```python
from build123d import *

# Parameters (mm, degrees)
SKETCH2_R           = 12.5
SKETCH2_R_2         = 11.5
SKETCH14_W          = 50
SKETCH14_H          = 23
BOSS_EXTRUDE1_DEPTH = 381.5
SKETCH15_R          = 6.5
CUT_EXTRUDE1_DEPTH  = 436.5
SKETCH16_W          = 40
SKETCH16_H          = 100
BOSS_EXTRUDE2_DEPTH = 5
SKETCH18_R          = 6.5
BOSS_EXTRUDE3_DEPTH = 10


with BuildPart() as part:
    # Sweep-Thin1: sweep along a path in Sketch1
    with BuildLine(Plane(origin=(0, 0, 0), x_dir=(1, 0, 0), z_dir=(0, 1, 0))) as sweep_thin1_path:
        Line((0, 395), (-610, 395))
        ThreePointArc((-610, 395), (-716.066017178, 351.066017178), (-760, 245))
        Line((-760, 245), (-760, -245))
        ThreePointArc((-760, -245), (-716.066017178, -351.066017178), (-610, -395))
        Line((-610, -395), (0, -395))
    # Sketch2 → Sweep-Thin1 (sweep)
    with BuildSketch(Plane(origin=(0, 0, 395), x_dir=(0, 0, -1), z_dir=(1, 0, 0))):
        with Locations((12.5, 0)):
            Circle(SKETCH2_R)
        with Locations((12.5, 0)):
            Circle(SKETCH2_R_2, mode=Mode.SUBTRACT)
    sweep(path=sweep_thin1_path.line)

    # Sketch14 → Boss-Extrude1 (add, symmetric)
    with BuildSketch(Plane.XY):
        with Locations((-75, 0)):
            Rectangle(SKETCH14_W, SKETCH14_H)
    extrude(amount=BOSS_EXTRUDE1_DEPTH, both=True)

    # Sketch15 → Cut-Extrude1 (cut, symmetric)
    with BuildSketch(Plane.XY):
        with Locations((-15, 0)):
            Circle(SKETCH15_R)
    extrude(amount=CUT_EXTRUDE1_DEPTH, both=True, mode=Mode.SUBTRACT)

    # Sketch16 → Boss-Extrude2 (add)
    with BuildSketch(Plane.XZ.offset(11.5)):
        with Locations((-75, -307.601020514)):
            Rectangle(SKETCH16_W, SKETCH16_H)
    extrude(amount=BOSS_EXTRUDE2_DEPTH)

    # Sketch18 → Boss-Extrude3 (add)
    with BuildSketch(Plane(origin=(0, 0, -317.601020514), x_dir=(-1, 0, 0), z_dir=(0, 0, -1))):
        with BuildLine():
            Line((90, -16.5), (60, -16.5))
            Line((60, -16.5), (198.241047903, -193.477674036))
            ThreePointArc((198.241047903, -193.477674036), (204.902077591, -197.247200167), (212.277594342, -195.202598394))
            Line((212.277594342, -195.202598394), (220.426068509, -188.837650874))
            ThreePointArc((220.426068509, -188.837650874), (224.214109013, -182.01512928), (221.946736533, -174.548197259))
            Line((221.946736533, -174.548197259), (90, -16.5))
        make_face()
        with Locations((204.040209344, -176.258653836)):
            Circle(SKETCH18_R, mode=Mode.SUBTRACT)
    boss_extrude3 = extrude(amount=BOSS_EXTRUDE3_DEPTH)

    # Mirror1: Boss-Extrude3 across plane
    add(boss_extrude3.mirror(Plane(origin=(0, 0, -302.601020514), x_dir=(1, 0, 0), z_dir=(0, 0, -1))))


solid = part.part
```
Geometry check sheet. Reference: the model listing, model coordinates, mm. A direction names the side the tool comes from. Coordinates: 2 decimals unless noted, no trailing zeros. Loops run counter-clockwise (first coordinate to the right, second up) from the corner with the lowest first, then second, coordinate; pieces in that order, holes last. Notation, with made-up numbers: (40, 4) - (68, 4) arc R25 cw to (68, 23) - close; hole circle Ø8 at (66, 13). An arc over 180 degrees is marked (long way). One line per item, written item: value. Start each with the question number.
(1) Material ranges on line 1 (Z direction, x = -277, y = 0); line 2 (Z direction, x = -90.5, y = -55); line 3 (Y direction, x = -244, z = -382), recorded low to high. Write a range as [from, to].
(2) Depth check by flat-ended pin: P1, Ø1.5, axis at x = -76, y = -13.5, coming from the -Z side; P2, Ø8, axis at x = -96.5, z = -251, coming from the -Y side; P3, Ø12, axis at x = -114, z = -280.5, coming from the +Y side. Enter the tip coordinate at first touch or a pass-through.
(3) Cross-section at C-C on x = -601. Enter the section's corners in (y, z).
(4) Cross-section at B-B on y = -112.5. Enter the section's corners in (x, z).
(5) Cross-section at D-D on y = -47. Enter the section's corners in (x, z), plus the area to 3 significant figures.
(6) Cross-section at A-A on z = -137. Enter the section's corners in (x, y).
(7) Mould release check, pull along Y, two halves, no side actions. Record for faces 1 (the cylindrical face through (-300.73, 0.51, 393.99)), 2 (the cylindrical face through (-309.27, 3.755, -370.577)), 3 (the flat face through (-148, -106, -317.601)): released by +Y, released by -Y, zero draft, split by the parting line, or undercut.
(8) Tool access check on faces 4 (the flat face through (-148, -106, -327.601)), 5 (the flat face through (-50, 0, 5)), 6 (the flat face through (-75, 11.5, 5)), 7 (the flat face through (-75, 0, -381.5)), 8 (the cylindrical face through (-300.73, 0.55, 394.988)). Record the directions out of +Z, -Z, +X, -X, +Y, -Y that give a thin tool (end or side, any length) a straight path to the whole face; none if there is none.
Results below:
1. line 1: z = [-395, -394], [-371, -370], [370, 371], [394, 395]
1. line 2: z = [-327.6, -317.6], [-287.6, -277.6]
1. line 3: y = [-12.49, -11.49], [11.49, 12.49]
2. P1: stops at z = -357.6
2. P2: stops at y = -11.5
2. P3: stops at y = -38.06
3. outline: circle Ø25 at (0, -382.5); circle Ø25 at (0, 382.5); hole circle Ø23 at (0, -382.5); hole circle Ø23 at (0, 382.5)
4. outline: (-170.15, -327.6) - (-134.99, -327.6) - (-134.99, -317.6) - (-170.15, -317.6) - close; (-170.15, -287.6) - (-134.99, -287.6) - (-134.99, -277.6) - (-170.15, -277.6) - close
5. outline: (-115.46, -327.6) - (-83.82, -327.6) - (-83.82, -317.6) - (-115.46, -317.6) - close; (-115.46, -287.6) - (-83.82, -287.6) - (-83.82, -277.6) - (-115.46, -277.6) - close
5. area: 633 mm2
6. outline: circle Ø25 at (-747.5, 0); (-100, -11.5) - (-50, -11.5) - (-50, 11.5) - (-100, 11.5) - close; hole circle Ø23 at (-747.5, 0)
7. face 1: undercut
7. face 2: split by the parting line
7. face 3: zero draft
8. face 4: -Z, +X, -X, -Y
8. face 5: +X, +Y, -Y
8. face 6: +X, +Y
8. face 7: +X
8. face 8: none
